Could you check a few things on this model? Use its own coordinates, in mm. Face numbers are marked on the shaded views. Give positions to 0.01 mm unless a question says otherwise; leave off trailing zeros. Write each loop counter-clockwise with the first axis right and the second up, starting at its lowest first coordinate (ties: lowest second). Pieces come first, ordered by that corner, then holes. Notation, with made-up numbers: (25.25, 24.5) - (67.25, 24.5) arc R30 cw to (67.25, 59.5) - close; hole circle Ø1 at (-1.75, 51). An arc over 180 degrees is marked (long way). Answer as CSV lines item,"result". Start each with the question number.
Q1. Imagine slicing it at B-B on x = 0. List the corners of the cut face in (y, z) for me, and give its area (3 significant figures).
Q2. Will these pins go through, and if not, where does the flat tip stop? pin 1 Ø1 at (x, y) = (-1.5, 1) entering from +Z; pin 2 Ø4.5 at (x, y) = (4.5, 12) entering from +Z.
Q3. We'd pull the mould along X, two halves only. Please class the marked faces 1, 2, 3 and 4: pulls with the +X half, pulls with the -X half, needs draft (parallel to the pull), parting line crosses it, or undercut.
Q4. Imagine slicing it at C-C on z = -17. List the corners of the cut face in (x, y) for me.
Q5. Imagine slicing it at D-D on y = 6.25. List the corners of the cut face in (x, z) for me.
Q6. If I drill on line 1 along Y through (x, z) = (-0.5, -6); line 2 along X through (y, z) = (7.25, -4); line 3 along X through (y, z) = (1.75, 36), over which ranges is the centre line in solid material (lowest first)?
Q7. Imagine slicing it at A-A on z = 11.5. List the corners of the cut face in (x, y) for me, and give its area (3 significant figures).
```python
from build123d import *

# Parameters (mm, degrees)
CROQUIS1_W              = 70
CROQUIS1_H              = 100
SALIENTE_EXTRUIR1_DEPTH = 15
CROQUIS2_W              = 30
CROQUIS2_H              = 13
CORTAR_EXTRUIR1_DEPTH   = 72
CORTAR_EXTRUIR2_DEPTH   = 72
CROQUIS4_W              = 9
CROQUIS4_H              = 1.6
CORTAR_EXTRUIR3_DEPTH   = 2
CROQUIS6_W              = 8.2
CROQUIS6_H              = 2
CORTAR_EXTRUIR4_DEPTH   = 94.926889384
CORTAR_EXTRUIR5_DEPTH   = 8.2
CROQUIS8_W              = 70
CROQUIS8_H              = 57
SALIENTE_EXTRUIR3_DEPTH = 2
CROQUIS9_W              = 20
CROQUIS9_H              = 15
SALIENTE_EXTRUIR4_DEPTH = 2
CROQUIS10_W             = 70
CROQUIS10_H             = 22.450330877
SALIENTE_EXTRUIR5_DEPTH = 2
CROQUIS12_W             = 70
CROQUIS12_H             = 26
CORTAR_EXTRUIR6_DEPTH   = 64.356136246


with BuildPart() as part:
    # Croquis1 → Saliente-Extruir1 (new body)
    with BuildSketch(Plane(origin=(0, 0, 0), x_dir=(1, 0, 0), z_dir=(0, 1, 0))):
        Rectangle(CROQUIS1_W, CROQUIS1_H)
    extrude(amount=SALIENTE_EXTRUIR1_DEPTH)

    # Croquis2 → Cortar-Extruir1 (cut)
    with BuildSketch(Plane.XY.offset(50)):
        with Locations((0, 8.5)):
            Rectangle(CROQUIS2_W, CROQUIS2_H)
    extrude(amount=-CORTAR_EXTRUIR1_DEPTH, mode=Mode.SUBTRACT)

    # Croquis3 → Cortar-Extruir2 (cut)
    with BuildSketch(Plane.XZ):
        with BuildLine():
            Line((-10, 50), (10, 50))
            ThreePointArc((10, 50), (0, 40), (-10, 50))
        make_face()
    extrude(amount=-CORTAR_EXTRUIR2_DEPTH, mode=Mode.SUBTRACT)

    # Croquis4 → Cortar-Extruir3 (cut)
    with BuildSketch(Plane(origin=(0, 2, 0), x_dir=(1, 0, 0), z_dir=(0, 1, 0))):
        with Locations((0, -35.061869007)):
            Rectangle(CROQUIS4_W, CROQUIS4_H)
    extrude(amount=-CORTAR_EXTRUIR3_DEPTH, mode=Mode.SUBTRACT)

    # Croquis6 → Cortar-Extruir4 (cut, through all)
    with BuildSketch(Plane(origin=(0, 0, 35.861869007), x_dir=(-1, 0, 0), z_dir=(0, 0, -1))):
        with Locations((0, 2)):
            Rectangle(CROQUIS6_W, CROQUIS6_H)
    extrude(amount=-CORTAR_EXTRUIR4_DEPTH, mode=Mode.SUBTRACT)

    # Croquis7 → Cortar-Extruir5 (cut)
    with BuildSketch(Plane(origin=(-4.1, 0, 0), x_dir=(0, 0, -1), z_dir=(1, 0, 0))):
        Polygon((-40.879144777, 0.510423286), (-35.861869007, 1), (-40.879144777, 1), align=None)
    extrude(amount=CORTAR_EXTRUIR5_DEPTH, mode=Mode.SUBTRACT)

    # Croquis8 → Saliente-Extruir3 (add)
    with BuildSketch(Plane(origin=(0, 15, 0), x_dir=(1, 0, 0), z_dir=(0, 1, 0))):
        with Locations((0, -21.5)):
            Rectangle(CROQUIS8_W, CROQUIS8_H)
        Polygon((15, 22), (35, 22), (35, 27.549669123), (-35, 27.549669123), (-35, 22), align=None)
    extrude(amount=SALIENTE_EXTRUIR3_DEPTH)

    # Croquis9 → Saliente-Extruir4 (add)
    with BuildSketch(Plane(origin=(0, 15, 0), x_dir=(1, 0, 0), z_dir=(0, 1, 0))):
        with Locations((-25, 14.5)):
            Rectangle(CROQUIS9_W, CROQUIS9_H)
        with Locations((25, 14.5)):
            Rectangle(CROQUIS9_W, CROQUIS9_H)
    extrude(amount=SALIENTE_EXTRUIR4_DEPTH)

    # Croquis10 → Saliente-Extruir5 (add)
    with BuildSketch(Plane(origin=(0, 15, 0), x_dir=(1, 0, 0), z_dir=(0, 1, 0))):
        with Locations((0, 38.774834562)):
            Rectangle(CROQUIS10_W, CROQUIS10_H)
    extrude(amount=SALIENTE_EXTRUIR5_DEPTH)

    # Croquis12 → Cortar-Extruir6 (cut, through all)
    with BuildSketch(Plane(origin=(0, 17, 0), x_dir=(1, 0, 0), z_dir=(0, 1, 0))):
        with Locations((0, 37)):
            Rectangle(CROQUIS12_W, CROQUIS12_H)
    extrude(amount=-CORTAR_EXTRUIR6_DEPTH, mode=Mode.SUBTRACT)


solid = part.part
```
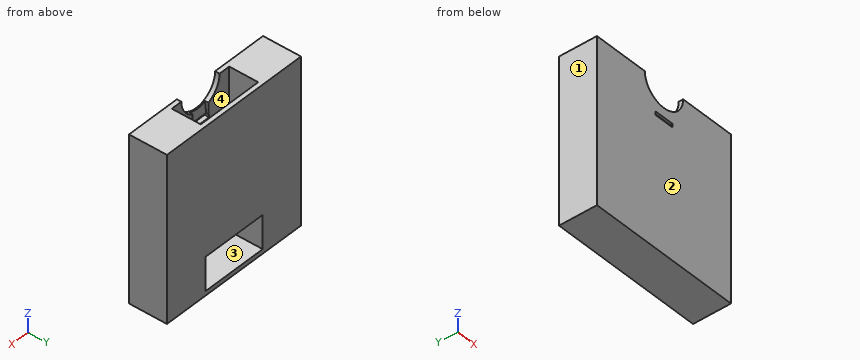
Conclusion:
1,outline,"(0, -24) - (17, -24) - (17, -22) - (2, -22) - (2, 34.26) - (0, 34.26) - close; (0, 35.86) - (1, 35.86) - (0.6, 40) - (0, 40) - close; (15, -7) - (17, -7) - (17, 50) - (15, 50) - close"
1,area,"264 mm^2"
2,pin 1,"z = 40.16"
2,pin 2,"z = -22"
3,face 1,"pulls with the -X half"
3,face 2,"needs draft"
3,face 3,"undercut"
3,face 4,"undercut"
4,outline,"(-35, 0) - (35, 0) - (35, 17) - (15, 17) - (15, 2) - (-15, 2) - (-15, 17) - (-35, 17) - close"
5,outline,"(-35, -24) - (35, -24) - (35, 50) - (15, 50) - (15, -22) - (-15, -22) - (-15, 50) - (-35, 50) - close"
6,line 1,"0 to 2, 15 to 17"
6,line 2,"-35 to -15, 15 to 35"
6,line 3,"-35 to -4.1, 4.1 to 35"
7,outline,"(-35, 0) - (35, 0) - (35, 17) - (-35, 17) - close; hole (-15, 2) - (15, 2) - (15, 15) - (-15, 15) - close"
7,area,"800 mm^2"
